Read the model definition and answer for the solid it produces. Units are mm, in the model's axes. A direction names the side the tool comes from. Coordinates: 2 decimals unless noted, no trailing zeros. Write each loop counter-clockwise with the first axis right and the second up, starting at its lowest first coordinate (ties: lowest second). Pieces come first, ordered by that corner, then holes.
1) The part is cut by section C-C (z = 24.5). Determine the outline of the cut face in (x, y).
2) Each of these flat-tipped pins is pushed along its axis until it touches: pin 1 Ø2 at (x, z) = (-8.5, 21.5) entering from +Y; pin 2 Ø1 at (x, z) = (-13.5, 7) entering from -Y; pin 3 Ø0.6 at (x, y) = (-9, -12) entering from -Z; pin 4 Ø4 at (x, z) = (-11, 23) entering from -Y. Where does it stop, or does it pass through?
3) Find the intervals of material crossed by line 1 (Y direction, x = -9.5, z = 21.85); line 2 (Y direction, x = -8.9, z = 6.15); line 3 (Z direction, x = -11.5, y = 4), in increasing order.
4) The part is cut by section D-D (y = -27). Determine the outline of the cut face in (x, z), then the cut area to 3 significant figures.
5) The part is cut by section A-A (z = 14). Determine the outline of the cut face in (x, y), then the cut area to 3 significant figures.
6) The part is cut by section B-B (x = -11). Determine the outline of the cut face in (y, z).
7) Which of the six approach directions +Z, -Z, +X, -X, +Y, -Y give full straight-line access (tool end or side, diameter ignored) to faces 1 (the face through (-9.876, 3.602, 17.043)), 2 (the face through (-9, -23, 3)), 3 (the face through (-16, 2.588, 14)), 4 (the face through (-9, -8, 25))?
8) Determine the mould class of faces 5 (the face through (-9, -22, 17)), 6 (the face through (-16.953, 5, 14)), 7 (the face through (-9, 2.588, 14)) for opening direction X: +X half, -X half, draft (parallel to the pull), parting line (faces both ways), or undercut.
from build123d import *

# Parameters (mm, degrees)
BOSS_EXTRUDE3_DEPTH = 28
SKETCH4_R           = 3.43
SKETCH4_R_2         = 1.5
CUT_EXTRUDE1_DEPTH  = 2
SKETCH6_W           = 3
SKETCH6_H           = 45
CUT_EXTRUDE4_DEPTH  = 2
SKETCH7_R           = 1.75
CUT_EXTRUDE5_DEPTH  = 3
SKETCH10_W          = 8
SKETCH10_H          = 14
CUT_EXTRUDE7_DEPTH  = 10


with BuildPart() as part:
    # Sketch3 → Boss-Extrude3 (new body)
    with BuildSketch(Plane.XY):
        Polygon((-16.953175304, 6.6875), (-14.953175304, 6.6875), (-14.953175304, 4.5875), (-7.953175304, 4.5875), (-7.953175304, -45.4125), (-9.953175304, -45.4125), (-9.953175304, 2.5875), (-16.953175304, 2.5875), align=None)
    extrude(amount=BOSS_EXTRUDE3_DEPTH)

    # Sketch4 → Cut-Extrude1 (cut)
    with BuildSketch(Plane(origin=(0, 4.5875, 0), x_dir=(1, 0, 0), z_dir=(0, 1, 0))):
        with Locations((-11.458423587, -14)):
            Circle(SKETCH4_R)
        with Locations((-11.383175304, -5.822)):
            Circle(SKETCH4_R_2)
        with Locations((-11.383175304, -22.177653801)):
            Circle(SKETCH4_R_2)
    extrude(amount=-CUT_EXTRUDE1_DEPTH, mode=Mode.SUBTRACT)

    # Sketch6 → Cut-Extrude4 (cut)
    with BuildSketch(Plane(origin=(-7.953175304, 0, 0), x_dir=(0, 0, -1), z_dir=(1, 0, 0))):
        with Locations((-26.5, -22.9125)):
            Rectangle(SKETCH6_W, SKETCH6_H)
        with Locations((-1.5, -22.9125)):
            Rectangle(SKETCH6_W, SKETCH6_H)
    extrude(amount=-CUT_EXTRUDE4_DEPTH, mode=Mode.SUBTRACT)

    # Sketch7 → Cut-Extrude5 (cut, through all)
    with BuildSketch(Plane.ZY.offset(9.953175304)):
        with Locations((21.85, -42.2625)):
            Circle(SKETCH7_R)
        with Locations((6.15, -42.2625)):
            Circle(SKETCH7_R)
        with Locations((6.15, -1.5625)):
            Circle(SKETCH7_R)
        with Locations((21.85, -1.5625)):
            Circle(SKETCH7_R)
    extrude(amount=-CUT_EXTRUDE5_DEPTH, mode=Mode.SUBTRACT)

    # Sketch10 → Cut-Extrude7 (cut, through all)
    with BuildSketch(Plane(origin=(-7.953175304, 0, 0), x_dir=(0, 0, -1), z_dir=(1, 0, 0))):
        with Locations((-21, -21.9125)):
            Rectangle(SKETCH10_W, SKETCH10_H)
    extrude(amount=-CUT_EXTRUDE7_DEPTH, mode=Mode.SUBTRACT)


solid = part.part
Reported:
1. outline: (-16.95, 2.59) - (-9.95, 2.59) - (-9.95, -14.91) - (-7.95, -14.91) - (-7.95, 4.59) - (-14.95, 4.59) - (-14.95, 6.69) - (-16.95, 6.69) - close; (-9.95, -45.41) - (-7.95, -45.41) - (-7.95, -28.91) - (-9.95, -28.91) - close
2. pin 1: stops at y = 4.59
2. pin 2: stops at y = 2.59
2. pin 3: stops at z = 3
2. pin 4: stops at y = -45.41
3. line 1: y = -45.41 to -44.01, -40.51 to -28.91, -14.91 to -3.31, 0.19 to 4.59
3. line 2: y = -45.41 to -44.01, -40.51 to -3.31, 0.19 to 4.59
3. line 3: z = 0 to 4.33, 7.32 to 10.57, 17.43 to 20.68, 23.67 to 28
4. outline: (-9.95, 3) - (-7.95, 3) - (-7.95, 17) - (-9.95, 17) - close
4. area: 28.0 mm2
5. outline: (-16.95, 2.59) - (-14.89, 2.59) - (-14.89, 4.59) - (-14.95, 4.59) - (-14.95, 6.69) - (-16.95, 6.69) - close; (-9.95, -45.41) - (-7.95, -45.41) - (-7.95, 4.59) - (-8.03, 4.59) - (-8.03, 2.59) - (-9.95, 2.59) - close
5. area: 104 mm2
6. outline: (2.59, 0) - (4.59, 0) - (4.59, 4.37) - (2.59, 4.37) - close; (2.59, 7.27) - (4.59, 7.27) - (4.59, 10.6) - (2.59, 10.6) - close; (2.59, 17.4) - (4.59, 17.4) - (4.59, 20.73) - (2.59, 20.73) - close; (2.59, 23.63) - (4.59, 23.63) - (4.59, 28) - (2.59, 28) - close
7. face 1: +Y
7. face 2: -Z, +X, -X, -Y
7. face 3: +Z, -Z, -X, -Y
7. face 4: +Z, +X, -X, -Y
8. face 5: draft
8. face 6: -X half
8. face 7: undercut
